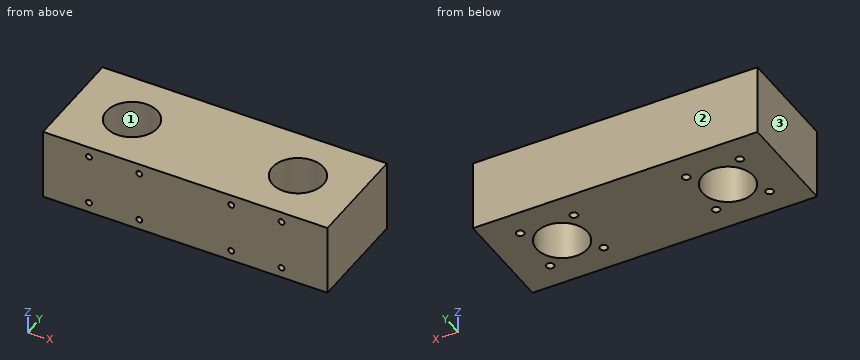
```python
from build123d import *

# Parameters (mm, degrees)
SKETCH_1_W             = 120
SKETCH_1_H             = 45
EXTRUDE_1_DEPTH        = 30
CUT_EXTRUDE_1_REACH    = 72.755
SKETCH_2_R             = 10.75
HOLE_WIZARD_M3_1_D     = 2.5
HOLE_WIZARD_M3_1_DEPTH = 7.5
HOLE_WIZARD_M3_1_TIP   = 0.751075774
HOLE_WIZARD_M4_1_D     = 3.3
HOLE_WIZARD_M4_1_DEPTH = 10.1
HOLE_WIZARD_M4_1_TIP   = 0.991420021


with BuildPart() as part:
    # 草图1 → 凸台-拉伸1 (new body)
    with BuildSketch(Plane.XY):
        Rectangle(SKETCH_1_W, SKETCH_1_H)
    extrude(amount=EXTRUDE_1_DEPTH)

    # 草图2 → 切除-拉伸1 (cut, up to next)
    with BuildSketch(Plane.XY.offset(30), mode=Mode.PRIVATE) as cut_extrude_1_sk1:
        with Locations((-35, 0)):
            Circle(SKETCH_2_R)
    cut_extrude_1_tool1 = extrude(cut_extrude_1_sk1.sketch, amount=-CUT_EXTRUDE_1_REACH, mode=Mode.PRIVATE) & part.part
    # 草图2 → 切除-拉伸1 (cut, up to next)
    with BuildSketch(Plane.XY.offset(30), mode=Mode.PRIVATE) as cut_extrude_1_sk2:
        with Locations((35, 0)):
            Circle(SKETCH_2_R)
    cut_extrude_1_tool2 = extrude(cut_extrude_1_sk2.sketch, amount=-CUT_EXTRUDE_1_REACH, mode=Mode.PRIVATE) & part.part
    add(cut_extrude_1_tool1.solids().sort_by_distance((-35, 0, 30))[0], mode=Mode.SUBTRACT)
    add(cut_extrude_1_tool2.solids().sort_by_distance((35, 0, 30))[0], mode=Mode.SUBTRACT)

    # M3 螺纹孔1
    with Locations(Plane(origin=(0, -22.5, 0), x_dir=(-1, 0, 0), z_dir=(0, -1, 0))):
        with Locations((-40.606601718, -4.393398282), (-19.393398282, -4.393398282), (-19.393398282, -25.606601718), (-40.606601718, -25.606601718), (19.393398282, -4.393398282), (40.606601718, -4.393398282), (19.393398282, -25.606601718), (40.606601718, -25.606601718)):
            Hole(HOLE_WIZARD_M3_1_D / 2, depth=HOLE_WIZARD_M3_1_DEPTH)
            with Locations((0, 0, -(HOLE_WIZARD_M3_1_DEPTH + HOLE_WIZARD_M3_1_TIP / 2))):  # 118° drill point
                Cone(0, HOLE_WIZARD_M3_1_D / 2, HOLE_WIZARD_M3_1_TIP, mode=Mode.SUBTRACT)

    # M4 螺纹孔1
    with Locations(Plane(origin=(-46.3, 11.3, 0), x_dir=(-1, 0, 0), z_dir=(0, 0, -1))):
        with Locations((0, 0), (0, -22.6), (-22.6, -22.6), (-22.6, 0), (-70, 0), (-70, -22.6), (-92.6, -22.6), (-92.6, 0)):
            Hole(HOLE_WIZARD_M4_1_D / 2, depth=HOLE_WIZARD_M4_1_DEPTH)
            with Locations((0, 0, -(HOLE_WIZARD_M4_1_DEPTH + HOLE_WIZARD_M4_1_TIP / 2))):  # 118° drill point
                Cone(0, HOLE_WIZARD_M4_1_D / 2, HOLE_WIZARD_M4_1_TIP, mode=Mode.SUBTRACT)


solid = part.part
```
Geometry check sheet. Reference: the model listing, model coordinates, mm. Face numbers are marked on the shaded views. Coordinates: 2 decimals unless noted, no trailing zeros. Write each loop counter-clockwise with the first axis right and the second up, starting at its lowest first coordinate (ties: lowest second). Pieces come first, ordered by that corner, then holes. Notation, with made-up numbers: M 66,-30 L 115,-30 A25 ccw 115,-16 Z; hole C 38,-27.5 d6. An arc over 180 degrees is marked long. One line per item, written item: value. Start each with the question number.
(1) Sectioned sample at A-A, the plane y = 0. Enter the section's corners in (x, z).
(2) Scan lines: line 1 along X through (y, z) = (11.3, 2.5); line 2 along Z through (x, y) = (40.5, -17.5); line 3 along Y through (x, z) = (46.3, 2.75). Record each from-to range of solid material in increasing order. Write a range as [from, to].
(3) Depth check by flat-ended pin: pin 1 (4 mm diameter, centred on x = 46.3, y = 11.3, fed in from -Z); pin 2 (2.5 mm diameter, centred on x = -23.7, y = -11.3, fed in from -Z). Enter the tip coordinate at first touch or a pass-through.
(4) Sectioned sample at B-B, the plane x = -35. Enter the section's corners in (y, z).
(5) Sectioned sample at D-D, the plane y = -6.5. Enter the section's corners in (x, z).
(6) Release check for a two-part mould opening along X. For the marked faces 1, 2 and 3 record: released by +X, released by -X, zero draft, split by the parting line, or undercut.
(7) Sectioned sample at C-C, the plane z = 18.75. Enter the section's corners in (x, y).
Filled sheet:
1. outline: M -60,0 L -45.75,0 L -45.75,30 L -60,30 Z; M -24.25,0 L 24.25,0 L 24.25,30 L -24.25,30 Z; M 45.75,0 L 60,0 L 60,30 L 45.75,30 Z
2. line 1: [-60, -47.95], [-44.65, -25.35], [-22.05, 22.05], [25.35, 44.65], [47.95, 60]
2. line 2: [0, 3.15], [5.64, 24.36], [26.85, 30]
2. line 3: [-22.5, -12.95], [-9.65, 9.65], [12.95, 22.5]
3. pin 1: z = 0
3. pin 2: z = 10.34
4. outline: M -22.5,0 L -10.75,0 L -10.75,30 L -22.5,30 Z; M 10.75,0 L 22.5,0 L 22.5,30 L 10.75,30 Z
5. outline: M -60,0 L -43.56,0 L -43.56,30 L -60,30 Z; M -26.44,0 L 26.44,0 L 26.44,30 L -26.44,30 Z; M 43.56,0 L 60,0 L 60,30 L 43.56,30 Z
6. face 1: undercut
6. face 2: zero draft
6. face 3: released by -X
7. outline: M -60,-22.5 L 60,-22.5 L 60,22.5 L -60,22.5 Z; hole C -35,0 d21.5; hole C 35,0 d21.5
